The listing builds one solid part. Answer for the finished solid, in the listing's coordinates (mm). A direction names the side the tool comes from. Give positions to 0.01 mm unless a question says otherwise; leave off trailing zeros. Loops run counter-clockwise (first coordinate to the right, second up) from the corner with the lowest first, then second, coordinate; pieces in that order, holes last. Notation, with made-up numbers: (82.25, 36.5) -> (117.25, 36.5) arc R21 cw to (117.25, 40.5) -> close; hole circle Ø5 at (4, 8). An arc over 180 degrees is marked (long way). One line per question, with ' | ' between items. Start each with the question number.
from build123d import *

# Parameters (mm, degrees)
SKETCH_1_W          = 80
SKETCH_1_H          = 80
SKETCH_1_W_2        = 70
SKETCH_1_H_2        = 70
EXTRUDE_1_DEPTH     = 5
SKETCH_2_W          = 5
SKETCH_2_H          = 5
EXTRUDE_2_DEPTH     = 75
SKETCH_4_W          = 5
SKETCH_4_H          = 5
EXTRUDE_3_DEPTH     = 70
EXTRUDE_4_DEPTH     = 5
SKETCH_7_W          = 5
SKETCH_7_H          = 5
EXTRUDE_5_DEPTH     = 70
EXTRUDE_6_DEPTH     = 5
SKETCH_11_R         = 2
SKETCH_11_R_2       = 1.5
EXTRUDE_7_DEPTH     = 1.5
CUT_EXTRUDE_START   = -3
SKETCH_11_2_R       = 1.5
CUT_EXTRUDE_1_DEPTH = 3
SKETCH_12_R         = 2
SKETCH_12_R_2       = 1.5
EXTRUDE_8_DEPTH     = 1.5
CUT_EXTRUDE_START_2 = -3.5
SKETCH_12_2_R       = 1.5
CUT_EXTRUDE_2_DEPTH = 3.5
SKETCH_13_R         = 2
SKETCH_13_R_2       = 1.5
EXTRUDE_9_DEPTH     = 1.5
SKETCH_13_2_R       = 1.5
CUT_EXTRUDE_3_DEPTH = 3


with BuildPart() as part:
    # 草图1 → 凸台-拉伸1 (new body)
    # profile 1 of 6: a face of its own
    with BuildSketch(Plane(origin=(0, 0, 0), x_dir=(1, 0, 0), z_dir=(0, 1, 0))):
        with Locations((40, 40)):
            Rectangle(SKETCH_1_W, SKETCH_1_H)
        with Locations((40, 40)):
            Rectangle(SKETCH_1_W_2, SKETCH_1_H_2, mode=Mode.SUBTRACT)
    # profile 2 of 6: a face of its own
    with BuildSketch(Plane(origin=(0, 0, 0), x_dir=(1, 0, 0), z_dir=(0, 1, 0))):
        Polygon((5, 8.535533906), (5, 5), (8.535533906, 5), (40, 36.464466094), (36.464466094, 40), align=None)
    # profile 3 of 6: a face of its own
    with BuildSketch(Plane(origin=(0, 0, 0), x_dir=(1, 0, 0), z_dir=(0, 1, 0))):
        Polygon((40, 36.464466094), (71.464466094, 5), (75, 5), (75, 8.535533906), (43.535533906, 40), align=None)
    # profile 4 of 6: a face of its own
    with BuildSketch(Plane(origin=(0, 0, 0), x_dir=(1, 0, 0), z_dir=(0, 1, 0))):
        Polygon((40, 43.535533906), (43.535533906, 40), (75, 71.464466094), (75, 75), (71.464466094, 75), align=None)
    # profile 5 of 6: a face of its own
    with BuildSketch(Plane(origin=(0, 0, 0), x_dir=(1, 0, 0), z_dir=(0, 1, 0))):
        Polygon((5, 75), (5, 71.464466094), (36.464466094, 40), (40, 43.535533906), (8.535533906, 75), align=None)
    # profile 6 of 6: a face of its own
    with BuildSketch(Plane(origin=(0, 0, 0), x_dir=(1, 0, 0), z_dir=(0, 1, 0))):
        Polygon((36.464466094, 40), (40, 36.464466094), (43.535533906, 40), (40, 43.535533906), align=None)
    extrude(amount=EXTRUDE_1_DEPTH)

    # 草图2 → 凸台-拉伸2 (add)
    with BuildSketch(Plane(origin=(0, 5, 0), x_dir=(1, 0, 0), z_dir=(0, 1, 0))):
        with Locations((2.5, 2.5)):
            Rectangle(SKETCH_2_W, SKETCH_2_H)
        with Locations((77.5, 2.5)):
            Rectangle(SKETCH_2_W, SKETCH_2_H)
        with Locations((2.5, 77.5)):
            Rectangle(SKETCH_2_W, SKETCH_2_H)
    extrude(amount=EXTRUDE_2_DEPTH)

    # 草图4 → 凸台-拉伸3 (add)
    with BuildSketch(Plane(origin=(5, 0, 0), x_dir=(0, 0, -1), z_dir=(1, 0, 0))):
        with Locations((2.5, 77.5)):
            Rectangle(SKETCH_4_W, SKETCH_4_H)
    extrude(amount=EXTRUDE_3_DEPTH)

    # 草图6 → 凸台-拉伸4 (add)
    with BuildSketch(Plane.XY):
        Polygon((5, 75), (5, 71.464466094), (36.464466094, 40), (40, 43.535533906), (8.535533906, 75), align=None)
        Polygon((40, 43.535533906), (43.535533906, 40), (75, 71.464466094), (75, 75), (71.464466094, 75), align=None)
        Polygon((5, 8.535533906), (5, 5), (8.535533906, 5), (40, 36.464466094), (36.464466094, 40), align=None)
        Polygon((36.464466094, 40), (40, 36.464466094), (43.535533906, 40), (40, 43.535533906), align=None)
        Polygon((40, 36.464466094), (71.464466094, 5), (75, 5), (75, 8.535533906), (43.535533906, 40), align=None)
    extrude(amount=-EXTRUDE_4_DEPTH)

    # 草图7 → 凸台-拉伸5 (add)
    with BuildSketch(Plane(origin=(0, 0, -5), x_dir=(-1, 0, 0), z_dir=(0, 0, -1))):
        with Locations((-2.5, 77.5)):
            Rectangle(SKETCH_7_W, SKETCH_7_H)
    extrude(amount=EXTRUDE_5_DEPTH)

    # 草图8 → 凸台-拉伸6 (add)
    with BuildSketch(Plane.ZY):
        Polygon((-5, 75), (-8.535533906, 75), (-40, 43.535533906), (-36.464466094, 40), (-5, 71.464466094), align=None)
        Polygon((-40, 43.535533906), (-43.535533906, 40), (-40, 36.464466094), (-36.464466094, 40), align=None)
        Polygon((-36.464466094, 40), (-40, 36.464466094), (-8.535533906, 5), (-5, 5), (-5, 8.535533906), align=None)
        Polygon((-71.464466094, 75), (-75, 75), (-75, 71.464466094), (-43.535533906, 40), (-40, 43.535533906), align=None)
        Polygon((-43.535533906, 40), (-75, 8.535533906), (-75, 5), (-71.464466094, 5), (-40, 36.464466094), align=None)
    extrude(amount=-EXTRUDE_6_DEPTH)

    # 草图11 → 凸台-拉伸7 (add)
    # profile 1 of 4: a face of its own
    with BuildSketch(Plane(origin=(0, 5, 0), x_dir=(1, 0, 0), z_dir=(0, 1, 0))):
        with Locations(Location((47, 47, 0), (0, 0, 270))):
            Circle(SKETCH_11_R)
        with Locations(Location((47, 47, 0), (0, 0, 270))):
            Circle(SKETCH_11_R_2, mode=Mode.SUBTRACT)
    # profile 2 of 4: a face of its own
    with BuildSketch(Plane(origin=(0, 5, 0), x_dir=(1, 0, 0), z_dir=(0, 1, 0))):
        with Locations(Location((47, 33, 0), (0, 0, 270))):
            Circle(SKETCH_11_R)
        with Locations(Location((47, 33, 0), (0, 0, 270))):
            Circle(SKETCH_11_R_2, mode=Mode.SUBTRACT)
    # profile 3 of 4: a face of its own
    with BuildSketch(Plane(origin=(0, 5, 0), x_dir=(1, 0, 0), z_dir=(0, 1, 0))):
        with Locations(Location((33, 33, 0), (0, 0, 270))):
            Circle(SKETCH_11_R)
        with Locations(Location((33, 33, 0), (0, 0, 270))):
            Circle(SKETCH_11_R_2, mode=Mode.SUBTRACT)
    # profile 4 of 4: a face of its own
    with BuildSketch(Plane(origin=(0, 5, 0), x_dir=(1, 0, 0), z_dir=(0, 1, 0))):
        with Locations(Location((33, 47, 0), (0, 0, 270))):
            Circle(SKETCH_11_R)
        with Locations(Location((33, 47, 0), (0, 0, 270))):
            Circle(SKETCH_11_R_2, mode=Mode.SUBTRACT)
    extrude(amount=EXTRUDE_7_DEPTH)

    # 草图11<2> → 切除-拉伸1 (cut)
    with BuildSketch(Plane(origin=(0, 5, 0), x_dir=(1, 0, 0), z_dir=(0, 1, 0)).offset(CUT_EXTRUDE_START)):
        with Locations(Location((33, 47, 0), (0, 0, 270))):
            Circle(SKETCH_11_2_R)
        with Locations(Location((33, 33, 0), (0, 0, 270))):
            Circle(SKETCH_11_2_R)
        Polygon((36, 39.535533906), (33.214466094, 36.75), (36, 36.75), align=None)
        Polygon((36, 43.25), (33.214466094, 43.25), (36, 40.464466094), align=None)
        Polygon((44, 40.464466094), (46.785533906, 43.25), (44, 43.25), align=None)
        Polygon((44, 36.75), (46.785533906, 36.75), (44, 39.535533906), align=None)
        with Locations(Location((47, 47, 0), (0, 0, 270))):
            Circle(SKETCH_11_2_R)
        with Locations(Location((47, 33, 0), (0, 0, 270))):
            Circle(SKETCH_11_2_R)
        with Locations(Location((40, 40, 0), (0, 0, 270))):
            Circle(SKETCH_11_2_R)
    extrude(amount=CUT_EXTRUDE_1_DEPTH, mode=Mode.SUBTRACT)

    # 草图12 → 凸台-拉伸8 (add)
    # profile 1 of 4: a face of its own
    with BuildSketch(Plane(origin=(0, 0, -5), x_dir=(-1, 0, 0), z_dir=(0, 0, -1))):
        with Locations(Location((-33, 47, 0), (0, 0, 180))):
            Circle(SKETCH_12_R)
        with Locations((-33, 47)):
            Circle(SKETCH_12_R_2, mode=Mode.SUBTRACT)
    # profile 2 of 4: a face of its own
    with BuildSketch(Plane(origin=(0, 0, -5), x_dir=(-1, 0, 0), z_dir=(0, 0, -1))):
        with Locations((-33, 33)):
            Circle(SKETCH_12_R)
        with Locations(Location((-33, 33, 0), (0, 0, 180))):
            Circle(SKETCH_12_R_2, mode=Mode.SUBTRACT)
    # profile 3 of 4: a face of its own
    with BuildSketch(Plane(origin=(0, 0, -5), x_dir=(-1, 0, 0), z_dir=(0, 0, -1))):
        with Locations(Location((-47, 33, 0), (0, 0, 180))):
            Circle(SKETCH_12_R)
        with Locations((-47, 33)):
            Circle(SKETCH_12_R_2, mode=Mode.SUBTRACT)
    # profile 4 of 4: a face of its own
    with BuildSketch(Plane(origin=(0, 0, -5), x_dir=(-1, 0, 0), z_dir=(0, 0, -1))):
        with Locations((-47, 47)):
            Circle(SKETCH_12_R)
        with Locations(Location((-47, 47, 0), (0, 0, 180))):
            Circle(SKETCH_12_R_2, mode=Mode.SUBTRACT)
    extrude(amount=EXTRUDE_8_DEPTH)

    # 草图12<2> → 切除-拉伸2 (cut)
    with BuildSketch(Plane(origin=(0, 0, -5), x_dir=(-1, 0, 0), z_dir=(0, 0, -1)).offset(CUT_EXTRUDE_START_2)):
        with Locations((-47, 33)):
            Circle(SKETCH_12_2_R)
        with Locations((-33, 33)):
            Circle(SKETCH_12_2_R)
        with Locations((-33, 47)):
            Circle(SKETCH_12_2_R)
        with Locations((-47, 47)):
            Circle(SKETCH_12_2_R)
        Polygon((-44, 43.25), (-46.785533906, 43.25), (-44, 40.464466094), align=None)
        Polygon((-44, 39.535533906), (-46.785533906, 36.75), (-44, 36.75), align=None)
        Polygon((-33.214466094, 36.75), (-36, 39.535533906), (-36, 36.75), align=None)
        Polygon((-33.214466094, 43.25), (-36, 43.25), (-36, 40.464466094), align=None)
        with Locations((-40, 40)):
            Circle(SKETCH_12_2_R)
    extrude(amount=CUT_EXTRUDE_2_DEPTH, mode=Mode.SUBTRACT)

    # 草图13 → 凸台-拉伸9 (add)
    # profile 1 of 4: a face of its own
    with BuildSketch(Plane(origin=(5, 0, 0), x_dir=(0, 0, -1), z_dir=(1, 0, 0))):
        with Locations((33, 47)):
            Circle(SKETCH_13_R)
        with Locations(Location((33, 47, 0), (0, 0, 180))):
            Circle(SKETCH_13_R_2, mode=Mode.SUBTRACT)
    # profile 2 of 4: a face of its own
    with BuildSketch(Plane(origin=(5, 0, 0), x_dir=(0, 0, -1), z_dir=(1, 0, 0))):
        with Locations(Location((47, 47, 0), (0, 0, 180))):
            Circle(SKETCH_13_R)
        with Locations((47, 47)):
            Circle(SKETCH_13_R_2, mode=Mode.SUBTRACT)
    # profile 3 of 4: a face of its own
    with BuildSketch(Plane(origin=(5, 0, 0), x_dir=(0, 0, -1), z_dir=(1, 0, 0))):
        with Locations(Location((33, 33, 0), (0, 0, 180))):
            Circle(SKETCH_13_R)
        with Locations((33, 33)):
            Circle(SKETCH_13_R_2, mode=Mode.SUBTRACT)
    # profile 4 of 4: a face of its own
    with BuildSketch(Plane(origin=(5, 0, 0), x_dir=(0, 0, -1), z_dir=(1, 0, 0))):
        with Locations((47, 33)):
            Circle(SKETCH_13_R)
        with Locations(Location((47, 33, 0), (0, 0, 180))):
            Circle(SKETCH_13_R_2, mode=Mode.SUBTRACT)
    extrude(amount=EXTRUDE_9_DEPTH)

    # 草图13<2> → 切除-拉伸3 (cut)
    with BuildSketch(Plane(origin=(5, 0, 0), x_dir=(0, 0, -1), z_dir=(1, 0, 0)).offset(CUT_EXTRUDE_START)):
        with Locations(Location((33, 33, 0), (0, 0, 180))):
            Circle(SKETCH_13_2_R)
        with Locations(Location((33, 47, 0), (0, 0, 180))):
            Circle(SKETCH_13_2_R)
        with Locations(Location((47, 47, 0), (0, 0, 180))):
            Circle(SKETCH_13_2_R)
        with Locations(Location((47, 33, 0), (0, 0, 180))):
            Circle(SKETCH_13_2_R)
        Polygon((36, 43.25), (33.214466094, 43.25), (36, 40.464466094), align=None)
        Polygon((36, 39.535533906), (33.214466094, 36.75), (36, 36.75), align=None)
        Polygon((46.785533906, 36.75), (44, 39.535533906), (44, 36.75), align=None)
        Polygon((46.785533906, 43.25), (44, 43.25), (44, 40.464466094), align=None)
        with Locations((40, 40)):
            Circle(SKETCH_13_2_R)
    extrude(amount=CUT_EXTRUDE_3_DEPTH, mode=Mode.SUBTRACT)


solid = part.part
1. Determine the mould class of faces 1 (the flat face through (2.465, 59.048, -55.512)), 2 (the flat face through (40, 2, -40)) for opening direction X: released by +X, released by -X, zero draft, split by the parting line, or undercut.
2. The part is cut by section A-A (y = 73). Write down the section's boundary in (x, z).
3. Straight lines are drawn through the part: L1, parallel to X at y = 43.5, z = -4; L2, parallel to Y at x = 3.65, z = -47. For each, find the intervals that lie inside material, in ascending order.
4. The part is cut by section B-B (z = -26). Write down the section's boundary in (x, y).
5. The part is cut by section C-C (x = 50.5). Write down the section's boundary in (y, z).
6. For faces 3 (the flat face through (45, 36.75, -3)), 4 (the cylindrical face through (6, 31, -47)), 5 (the flat face through (59.488, 24.048, -2.465)), determine the directions among +Z, -Z, +X, -X, +Y, -Y from which every point of the face is accessible in a straight line to the end or side of a thin tool.
7. Each of these flat-tipped pins is pushed along its axis until it touches: pin 1 Ø12 at (x, y) = (14, 52.5) entering from -Z; pin 2 Ø1.2 at (y, z) = (33.5, -48) entering from +X; pin 3 Ø10 at (x, z) = (39, -35.5) entering from +Y; pin 4 Ø1.8 at (x, z) = (40, -40) entering from +Y. Where does it stop, or does it pass through?
Check sheet entries:
1) face 1: zero draft | face 2: undercut
2) outline: (0, -80) -> (5, -80) -> (5, -69.46) -> (0, -69.46) -> close; (0, -10.54) -> (5, -10.54) -> (5, -5) -> (10.54, -5) -> (10.54, 0) -> (0, 0) -> close; (69.46, -5) -> (80, -5) -> (80, 0) -> (69.46, 0) -> close
3) L1: x = 0 to 5, 32.96 to 47.04, 75 to 80 | L2: y = 0 to 5, 29.46 to 31.5, 34.5 to 36.54, 43.46 to 45.5, 48.5 to 50.54, 75 to 80
4) outline: (0, 0) -> (5, 0) -> (5, 5) -> (0, 5) -> close; (0, 22.46) -> (5, 22.46) -> (5, 29.54) -> (0, 29.54) -> close; (0, 50.46) -> (5, 50.46) -> (5, 57.54) -> (0, 57.54) -> close; (0, 75) -> (5, 75) -> (5, 80) -> (0, 80) -> close; (22.46, 0) -> (29.54, 0) -> (29.54, 5) -> (22.46, 5) -> close; (50.46, 0) -> (57.54, 0) -> (57.54, 5) -> (50.46, 5) -> close; (75, 0) -> (80, 0) -> (80, 5) -> (75, 5) -> close
5) outline: (0, -80) -> (5, -80) -> (5, -75) -> (0, -75) -> close; (0, -54.04) -> (5, -54.04) -> (5, -46.96) -> (0, -46.96) -> close; (0, -33.04) -> (5, -33.04) -> (5, -25.96) -> (0, -25.96) -> close; (0, -5) -> (5, -5) -> (5, 0) -> (0, 0) -> close; (25.96, -5) -> (33.04, -5) -> (33.04, 0) -> (25.96, 0) -> close; (46.96, -5) -> (54.04, -5) -> (54.04, 0) -> (46.96, 0) -> close; (75, -5) -> (80, -5) -> (80, 0) -> (75, 0) -> close
6) face 3: -Z | face 4: +X | face 5: +Z, -Z
7) pin 1: passes through | pin 2: stops at x = 6.5 | pin 3: stops at y = 6.5 | pin 4: stops at y = 2
